from build123d import *

# Parameters (mm, degrees)
CROQUIS1_R                        = 7.5
SALIENTE_EXTRUIR1_DEPTH           = 10
CROQUIS2_R                        = 20
SALIENTE_EXTRUIR2_DEPTH           = 25
SALIENTE_EXTRUIR2_TAPER           = 30
CROQUIS3_R                        = 4
CORTAR_EXTRUIR2_DEPTH             = 70
TALADRO_DE_MARGEN_PARA_M41_REACH  = 47.571
TALADRO_DE_MARGEN_PARA_M41_BORE_R = 2.25


with BuildPart() as part:
    # Croquis1 → Saliente-Extruir1 (new body)
    with BuildSketch(Plane(origin=(0, 0, 0), x_dir=(0, 0, -1), z_dir=(1, 0, 0))):
        Circle(CROQUIS1_R)
    extrude(amount=SALIENTE_EXTRUIR1_DEPTH)

    # Croquis2 → Saliente-Extruir2 (add)
    with BuildSketch(Plane(origin=(10, 0, 0), x_dir=(0, 0, -1), z_dir=(1, 0, 0))):
        Circle(CROQUIS2_R)
    extrude(amount=SALIENTE_EXTRUIR2_DEPTH, taper=SALIENTE_EXTRUIR2_TAPER)

    # Croquis3 → Cortar-Extruir2 (cut)
    with BuildSketch(Plane(origin=(35, 0, 0), x_dir=(0, 0, -1), z_dir=(1, 0, 0))):
        Circle(CROQUIS3_R)
    extrude(amount=-CORTAR_EXTRUIR2_DEPTH, mode=Mode.SUBTRACT)

    # Taladro de margen para M41 bore (on position points) → Taladro de margen para M41 (cut, up to next)
    with BuildSketch(Plane(origin=(5, 7.481198926, -0.530718977), x_dir=(0, 0.070762530204, 0.997493190112), z_dir=(0, 0.997493190112, -0.070762530204)), mode=Mode.PRIVATE) as taladro_de_margen_para_m41_sk1:
        Circle(TALADRO_DE_MARGEN_PARA_M41_BORE_R)
    taladro_de_margen_para_m41_tool1 = extrude(taladro_de_margen_para_m41_sk1.sketch, amount=-TALADRO_DE_MARGEN_PARA_M41_REACH, mode=Mode.PRIVATE) & part.part
    add(taladro_de_margen_para_m41_tool1.solids().sort_by_distance((5, 7.481199, -0.530719))[0], mode=Mode.SUBTRACT)


solid = part.part
Could you check a few things on this model? Use its own coordinates, in mm. A direction names the side the tool comes from. Round coordinates to 2 decimals unless told otherwise and drop trailing zeros. Write each loop counter-clockwise with the first axis right and the second up, starting at its lowest first coordinate (ties: lowest second). Pieces come first, ordered by that corner, then holes. Notation, with made-up numbers: (81, 2) - (87, 2) arc R8 cw to (87, 17) - close; hole circle Ø4 at (31, 67). An arc over 180 degrees is marked (long way). Use a Markdown table: item, result.
Q1. I want a section at C-C (x = 31). List the corners of the cut face in (y, z) for me, plus the area to 3 significant figures.
Output values:
| item | result |
|---|---|
| outline | circle Ø15.75 at (0, 0); hole circle Ø8 at (0, 0) |
| area | 145 mm2 |
Q2. For pin 1 (3 mm diameter, centred on y = 0, z = -13.5, fed in from +X); pin 2 (3 mm diameter, centred on x = 26.5, z = 2, fed in from -Y); pin 3 (8 mm diameter, centred on x = 17, z = -0.5, fed in from -Y), each with a flat end and sliding along its axis, tell me the tip position at first contact or that it passes through.
Output values:
| item | result |
|---|---|
| pin 1 | x = 23.86 |
| pin 2 | y = -11.19 |
| pin 3 | y = -18.26 |
Q3. I want a section at A-A (x = 8). List the corners of the cut face in (y, z) for me.
Output values:
| item | result |
|---|---|
| outline | circle Ø15 at (0, 0); hole circle Ø8 at (0, 0) |
Q4. Please list where these lines run through material, in increasing order: L1, parallel to Z at x = 26.5, y = 3; L2, parallel to Z at x = 25, y = -1; L3, parallel to Y at x = 13, z = -3.5.
Output values:
| item | result |
|---|---|
| L1 | -10.03 to -2.65, 2.65 to 10.03 |
| L2 | -11.3 to -3.87, 3.87 to 11.3 |
| L3 | -17.93 to -1.94, 1.94 to 17.93 |
Q5. For faces 4 (the cylindrical face through (17.745, -3.905, 0.867)), 5 (the flat face through (10, 0, -9)), which set-ups out of +Z, -Z, +X, -X, +Y, -Y let a thin tool reach every point of the face, with its end or its side?
Output values:
| item | result |
|---|---|
| face 4 | +X, -X |
| face 5 | -X |
Q6. Thinking about a two-plate mould opening in Y: for faces 1 (the cylindrical face through (4.93, -7.32, 1.63)), 2 (the flat face through (0, -3, -3)), 3 (the cylindrical face through (5.676, 5.572, 1.756)), which applies, released by +Y, released by -Y, zero draft, split by the parting line, or undercut?
Output values:
| item | result |
|---|---|
| face 1 | split by the parting line |
| face 2 | zero draft |
| face 3 | undercut |
Q7. I want a section at B-B (z = 0). Count the separate pieces of the cut face and the enclosed holes in it, plus the area to 3 significant figures.
Output values:
| item | result |
|---|---|
| separate pieces | 3 |
| enclosed holes | 0 |
| area | 494 mm2 |
